from build123d import *

# Parameters (mm, degrees)
BOSS_EXTRU_1_DEPTH      = 300
ESQUISSE2_R             = 2
ENL_V_MAT_EXTRU_1_DEPTH = 301.333148354


with BuildPart() as part:
    # Esquisse1 → Boss.-Extru.1 (new body)
    with BuildSketch(Plane.XY):
        with BuildLine():
            Line((2, 0), (8, 0))
            ThreePointArc((8, 0), (9.414213562, 0.585786438), (10, 2))
            Line((10, 2), (10, 8))
            ThreePointArc((10, 8), (9.414213562, 9.414213562), (8, 10))
            Line((8, 10), (2, 10))
            ThreePointArc((2, 10), (0.585786438, 9.414213562), (0, 8))
            Line((0, 8), (0, 2))
            ThreePointArc((0, 2), (0.585786438, 0.585786438), (2, 0))
        make_face()
        with BuildLine():
            Line((3, 8), (7, 8))
            ThreePointArc((7, 8), (7.707106781, 7.707106781), (8, 7))
            Line((8, 7), (8, 3))
            ThreePointArc((8, 3), (7.707106781, 2.292893219), (7, 2))
            Line((7, 2), (3, 2))
            ThreePointArc((3, 2), (2.292893219, 2.292893219), (2, 3))
            Line((2, 3), (2, 7))
            ThreePointArc((2, 7), (2.292893219, 7.707106781), (3, 8))
        make_face(mode=Mode.SUBTRACT)
    extrude(amount=BOSS_EXTRU_1_DEPTH)

    # Esquisse2 → Enlèv. mat.-Extru.1 (cut, through all)
    with BuildSketch(Plane(origin=(0, 10, 0), x_dir=(1, 0, 0), z_dir=(0, 1, 0))):
        with Locations(Location((5, -294, 0), (0, 0, 270))):
            Circle(ESQUISSE2_R)
        with Locations(Location((5, -264, 0), (0, 0, 270))):
            Circle(ESQUISSE2_R)
        with Locations(Location((5, -7, 0), (0, 0, 270))):
            Circle(ESQUISSE2_R)
        with Locations(Location((5, -37, 0), (0, 0, 270))):
            Circle(ESQUISSE2_R)
    extrude(amount=-ENL_V_MAT_EXTRU_1_DEPTH, mode=Mode.SUBTRACT)


solid = part.part
Could you check a few things on this model? Use its own coordinates, in mm. Give positions to 0.01 mm unless a question says otherwise; leave off trailing zeros. Order: outer loops, then holes, each group sorted by start corner. A loop starts at its lowest first (then second) coordinate and runs counter-clockwise, first axis right, second up.
1. Suppose I cut it at C-C (x = 5). Give the number of separate pieces and of enclosed holes in the cut face, plus the area to 3 significant figures.
2. I need wall thicknesses on L1, parallel to Z at x = 5, y = 1.2; L2, parallel to Y at x = 3.75, z = 31.5; L3, parallel to X at y = 2.75, z = 216. Which ranges of each line are inside material? Lowest first, please.
3. Suppose I cut it at B-B (z = 119). List the corners of the cut face in (x, y) for me, plus the area to 3 significant figures.
4. Will this pin go through, and if not, where does the flat tip stop? P1, Ø2.5, axis at x = 5, z = 37, coming from the -Y side.
5. Suppose I cut it at A-A (y = 5.25). List the corners of the cut face in (x, z) for me, plus the area to 3 significant figures.
Solved:
1. separate pieces: 10
1. enclosed holes: 0
1. area: 1,140 mm2
2. L1: z = 0 to 5, 9 to 35, 39 to 262, 266 to 292, 296 to 300
2. L2: y = 0 to 2, 8 to 10
2. L3: x = 0 to 2.03, 7.97 to 10
3. outline: (0, 2) arc R2 ccw to (2, 0) - (8, 0) arc R2 ccw to (10, 2) - (10, 8) arc R2 ccw to (8, 10) - (2, 10) arc R2 ccw to (0, 8) - close; hole (2, 3) arc R1 ccw to (3, 2) - (7, 2) arc R1 ccw to (8, 3) - (8, 7) arc R1 ccw to (7, 8) - (3, 8) arc R1 ccw to (2, 7) - close
3. area: 61.4 mm2
4. P1: passes through
5. outline: (0, 0) - (2, 0) - (2, 300) - (0, 300) - close; (8, 0) - (10, 0) - (10, 300) - (8, 300) - close
5. area: 1,200 mm2
